Design review of the part built by this model. Coordinates are the model's own, in mm. A direction names the side the tool comes from. Coordinates: 2 decimals unless noted, no trailing zeros. Write each loop counter-clockwise with the first axis right and the second up, starting at its lowest first coordinate (ties: lowest second). Pieces come first, ordered by that corner, then holes. Notation, with made-up numbers: (-39, 1.5) -> (-29, 1.5) arc R19 ccw to (-29, 9.5) -> close; hole circle Ø8 at (23.25, 7.5). An arc over 180 degrees is marked (long way). Answer in a Markdown table with one row per item. Add a question column.
Item 1: Clearance check with a flat-ended pin moving along its axis: P1, Ø4, axis at y = 0, z = 0, coming from the -X side. State where the tip first meets the part, or that it passes through.
Item 2: Take a section at A-A, the plane x = 1.1. Write out the cut boundary in (y, z), and give its area (3 significant figures).
Item 3: To check wall thickness, follow line 1 (Y direction, x = 1.95, z = 0); line 2 (X direction, y = 2.5, z = 1.75); line 3 (Y direction, x = 0.5, z = -1). State the ranges of each line that lie inside material, in increasing order.
Item 4: For faces 1 (the face through (1.23, -2.44, 0.54)), 2 (the face through (2.3, 1, -3)), list the 3-axis set-ups (+Z, -Z, +X, -X, +Y, -Y) from which the entire face can be reached by the end or side of a thin tool; tool diameter is ignored.
Item 5: Draft analysis for pull direction Z (two halves, no side actions). For faces 3 (the face through (0.2, -1, -3)), 4 (the face through (1.234, -3.905, 0.867)), state which applies: released by +Z, released by -Z, zero draft, split by the parting line, or undercut.
from build123d import *

# Parameters (mm, degrees)
SKETCH_1_R          = 4
SKETCH_1_R_2        = 2.5
EXTRUDE_1_DEPTH     = 2.5
SKETCH_2_R          = 3.5
SKETCH_2_R_2        = 2.999624375
CUT_EXTRUDE_1_DEPTH = 0.2
SKETCH_3_R          = 3.5
SKETCH_3_R_2        = 2.950876812
CUT_EXTRUDE_2_DEPTH = 0.2
CHAMFER_1_SIZE      = 0.1


with BuildPart() as part:
    # 草图1 → 凸台-拉伸1 (new body)
    with BuildSketch(Plane(origin=(0, 0, 0), x_dir=(0, 0, -1), z_dir=(1, 0, 0))):
        Circle(SKETCH_1_R)
        Circle(SKETCH_1_R_2, mode=Mode.SUBTRACT)
    extrude(amount=EXTRUDE_1_DEPTH)

    # 草图2 → 切除-拉伸1 (cut)
    with BuildSketch(Plane(origin=(2.5, 0, 0), x_dir=(0, 0, -1), z_dir=(1, 0, 0))):
        with Locations((-0.000375625, 0)):
            Circle(SKETCH_2_R)
        with Locations((-0.000375625, 0)):
            Circle(SKETCH_2_R_2, mode=Mode.SUBTRACT)
    extrude(amount=-CUT_EXTRUDE_1_DEPTH, mode=Mode.SUBTRACT)

    # 草图3 → 切除-拉伸2 (cut)
    with BuildSketch(Plane.ZY):
        with Locations((-0.049123188, 0)):
            Circle(SKETCH_3_R)
        with Locations((-0.049123188, 0)):
            Circle(SKETCH_3_R_2, mode=Mode.SUBTRACT)
    extrude(amount=-CUT_EXTRUDE_2_DEPTH, mode=Mode.SUBTRACT)

    # 倒角1
    chamfer_1_edges = [part.edges().sort_by_distance(p)[0] for p in [
        (2.5, 0, 3.500375625),
        (0, 0, 4),
        (0, 0, -3.549123188),
        (0, 0, -3),
        (2.5, 0, 4),
        (0, 0, 2.5),
        (2.5, 0, 2.5),
    ]]
    chamfer(chamfer_1_edges, length=CHAMFER_1_SIZE)


solid = part.part
Answers:
| question | item | result |
|---|---|---|
| 1 | P1 | passes through |
| 2 | outline | circle Ø8 at (0, 0); hole circle Ø5 at (0, 0) |
| 2 | area | 30.6 mm^2 |
| 3 | line 1 | y = -4 to -2.5, 2.5 to 4 |
| 3 | line 2 | x = 0.2 to 2.3 |
| 3 | line 3 | y = -3.87 to -2.29, 2.29 to 3.87 |
| 4 | face 1 | +X, -X |
| 4 | face 2 | +X |
| 5 | face 3 | undercut |
| 5 | face 4 | split by the parting line |
